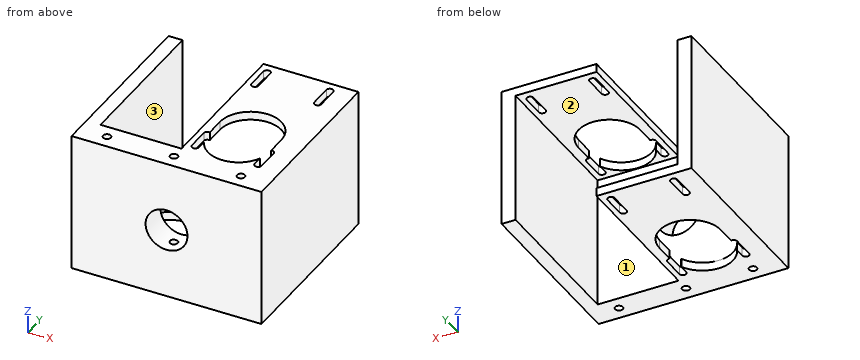
from build123d import *

# Parameters (mm, degrees)
BOSS_EXTRUDE1_DEPTH      = 25
BOSS_EXTRUDE1_DEPTH_BACK = 25
SKETCH1_W                = 5
SKETCH1_H                = 55
SKETCH1_W_2              = 68
SKETCH1_H_2              = 10
SKETCH2_W                = 29
SKETCH2_H                = 3
BOSS_EXTRUDE2_DEPTH      = 55
SKETCH4_R                = 7.5
CUT_EXTRUDE2_DEPTH       = 12
SKETCH6_R                = 1.375
CUT_EXTRUDE4_DEPTH       = 70
CUT_EXTRUDE11_DEPTH      = 61
SKETCH9_W                = 22
SKETCH9_H                = 5.846779426
CUT_EXTRUDE12_DEPTH      = 70


with BuildPart() as part:
    # Sketch1 → Boss-Extrude1 (new, two sides: drawn at the far end of the back side and taken through both)
    with BuildSketch(Plane.XY.offset(-BOSS_EXTRUDE1_DEPTH_BACK)):
        with Locations((-31.5, 32.5)):
            Rectangle(SKETCH1_W, SKETCH1_H)
        Rectangle(SKETCH1_W_2, SKETCH1_H_2)
        with Locations((31.5, 32.5)):
            Rectangle(SKETCH1_W, SKETCH1_H)
    extrude(amount=BOSS_EXTRUDE1_DEPTH + BOSS_EXTRUDE1_DEPTH_BACK)

    # Sketch2 → Boss-Extrude2 (add)
    with BuildSketch(Plane(origin=(0, 5, 0), x_dir=(1, 0, 0), z_dir=(0, 1, 0))):
        with Locations((14.5, -23.5)):
            Rectangle(SKETCH2_W, SKETCH2_H)
        with Locations((-14.5, 23.5)):
            Rectangle(SKETCH2_W, SKETCH2_H)
    extrude(amount=BOSS_EXTRUDE2_DEPTH)

    # Sketch4 → Cut-Extrude2 (cut)
    with BuildSketch(Plane(origin=(0, 5, 0), x_dir=(1, 0, 0), z_dir=(0, 1, 0))):
        with Locations(Location((0, 0, 0), (0, 0, 180))):
            Circle(SKETCH4_R)
    extrude(amount=-CUT_EXTRUDE2_DEPTH, mode=Mode.SUBTRACT)

    # Sketch6 → Cut-Extrude4 (cut)
    with BuildSketch(Plane.XY.offset(25)):
        Circle(SKETCH6_R)
        with Locations((24, 0)):
            Circle(SKETCH6_R)
        with Locations((-24, 0)):
            Circle(SKETCH6_R)
    extrude(amount=-CUT_EXTRUDE4_DEPTH, mode=Mode.SUBTRACT)

    # Sketch3 → Cut-Extrude11 (cut)
    with BuildSketch(Plane(origin=(0, 0, -25), x_dir=(-1, 0, 0), z_dir=(0, 0, -1))):
        with BuildLine():
            Line((25.5, 17.474744871), (25.5, 24.25))
            ThreePointArc((25.5, 24.25), (14.5, 35.25), (3.5, 24.25))
            Line((3.5, 24.25), (3.5, 17.474744871))
            ThreePointArc((3.5, 17.474744871), (2.459430585, 17.218245837), (2, 16.25))
            Line((2, 16.25), (2, 8.25))
            ThreePointArc((2, 8.25), (3.25, 7), (4.5, 8.25))
            Line((4.5, 8.25), (4.5, 11.667424305))
            ThreePointArc((4.5, 11.667424305), (14.5, 5.25), (24.5, 11.667424305))
            Line((24.5, 11.667424305), (24.5, 8.25))
            ThreePointArc((24.5, 8.25), (25.75, 7), (27, 8.25))
            Line((27, 8.25), (27, 16.25))
            ThreePointArc((27, 16.25), (26.540569415, 17.218245837), (25.5, 17.474744871))
        make_face()
        with BuildLine():
            Line((4.5, 48.25), (4.5, 56.25))
            ThreePointArc((4.5, 56.25), (3.25, 57.5), (2, 56.25))
            Line((2, 56.25), (2, 48.25))
            ThreePointArc((2, 48.25), (3.25, 47), (4.5, 48.25))
        make_face()
        with BuildLine():
            Line((27, 48.25), (27, 56.25))
            ThreePointArc((27, 56.25), (25.75, 57.5), (24.5, 56.25))
            Line((24.5, 56.25), (24.5, 48.25))
            ThreePointArc((24.5, 48.25), (25.75, 47), (27, 48.25))
        make_face()
    cut_extrude11 = extrude(amount=-CUT_EXTRUDE11_DEPTH, mode=Mode.SUBTRACT)

    # Sketch9 → Cut-Extrude12 (cut)
    with BuildSketch(Plane(origin=(0, 0, -25), x_dir=(-1, 0, 0), z_dir=(0, 0, -1))):
        with Locations((14.5, 14.551355158)):
            Rectangle(SKETCH9_W, SKETCH9_H)
    extrude(amount=-CUT_EXTRUDE12_DEPTH, mode=Mode.SUBTRACT)

    # Mirror3: Cut-Extrude11 across plane
    add(cut_extrude11.mirror(Plane(origin=(0, 0, 0), x_dir=(0, 0, 1), z_dir=(1, 0, 0))), mode=Mode.SUBTRACT)


solid = part.part
Verification items for the finished model (mm, model axes). Face numbers are marked on the shaded views. A direction names the side the tool comes from. Round coordinates to 2 decimals unless told otherwise and drop trailing zeros. Loops run counter-clockwise (first coordinate to the right, second up) from the corner with the lowest first, then second, coordinate; pieces in that order, holes last. Notation, with made-up numbers: (-10, 25.25) - (44, 25.25) arc R25 cw to (44, 39.25) - close; hole circle Ø1 at (-12, 47). An arc over 180 degrees is marked (long way). Answer in a Markdown table with one row per item. Add a question column.
Q1. Section check C-C on y = 23. Enter the section's corners in (x, z).
Q2. Tool access check on the marked faces 1, 2 and 3. Record the directions out of +Z, -Z, +X, -X, +Y, -Y that give a thin tool (end or side, any length) a straight path to the whole face; none if there is none.
Q3. Material ranges on line 1 (X direction, y = 52, z = -18); line 2 (X direction, y = 0.5, z = 19.5); line 3 (X direction, y = -1, z = -18), recorded low to high.
Q4. Section check B-B on x = 14.5. Enter the section's corners in (y, z).
Q5. Section check D-D on z = 11.5. Enter the section's corners in (x, y) (3 decimals), plus the area to 3 significant figures.
Q6. Gauge pin test, flat ends, axial feed: pin 1 (1 mm diameter, centred on x = 24.5, y = 49.5, fed in from -Z); pin 2 (12 mm diameter, centred on x = 0, z = 0, fed in from +Y); pin 3 (8 mm diameter, centred on x = 23.5, z = -16, fed in from +Y). Record the tip position at first contact, or that the pin passes through.
Q7. Section check A-A on y = 52. Enter the section's corners in (x, z).
Found:
| question | item | result |
|---|---|---|
| 1 | outline | (-34, -25) - (-25.5, -25) - (-25.5, -22) - (-29, -22) - (-29, 25) - (-34, 25) - close; (-3.5, -25) - (0, -25) - (0, -22) - (-3.5, -22) - close; (0, 22) - (3.5, 22) - (3.5, 25) - (0, 25) - close; (25.5, 22) - (29, 22) - (29, -25) - (34, -25) - (34, 25) - (25.5, 25) - close |
| 2 | face 1 | +Y |
| 2 | face 2 | -Z, +Y |
| 2 | face 3 | +Z, +Y |
| 3 | line 1 | x = -34 to -29, 29 to 34 |
| 3 | line 2 | x = -34 to -25.28, -22.72 to -1.28, 1.28 to 22.72, 25.28 to 34 |
| 3 | line 3 | x = -34 to -24.94, -23.06 to -0.94, 0.94 to 23.06, 24.94 to 34 |
| 4 | outline | (-5, -25) - (5, -25) - (5, 22) - (5.25, 22) - (5.25, 25) - (-5, 25) - close; (35.25, 22) - (60, 22) - (60, 25) - (35.25, 25) - close |
| 5 | outline | (-34, -5) - (34, -5) - (34, 60) - (29, 60) - (29, 5) - (-29, 5) - (-29, 60) - (-34, 60) - close; hole circle Ø2.75 at (-24, 0); hole circle Ø2.75 at (0, 0); hole circle Ø2.75 at (24, 0) |
| 5 | area | 1,210 mm² |
| 6 | pin 1 | stops at z = 22 |
| 6 | pin 2 | passes through |
| 6 | pin 3 | stops at y = 5 |
| 7 | outline | (-34, -25) - (-27, -25) - (-27, -22) - (-29, -22) - (-29, 25) - (-34, 25) - close; (-24.5, -25) - (-4.5, -25) - (-4.5, -22) - (-24.5, -22) - close; (-2, -25) - (0, -25) - (0, -22) - (-2, -22) - close; (0, 22) - (2, 22) - (2, 25) - (0, 25) - close; (4.5, 22) - (24.5, 22) - (24.5, 25) - (4.5, 25) - close; (27, 22) - (29, 22) - (29, -25) - (34, -25) - (34, 25) - (27, 25) - close |
